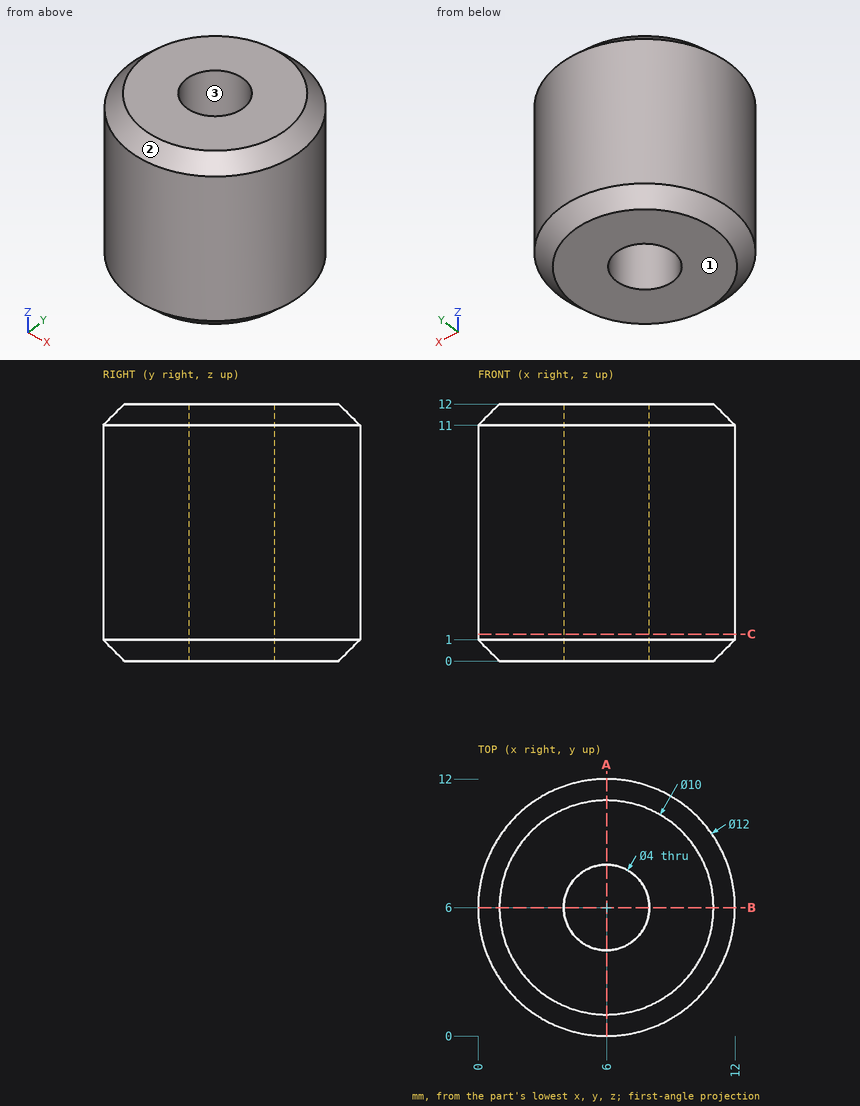
Study the drawing (mm; zero at the part's minimum x, y, z) and answer. Coordinates: 2 decimals unless noted, no trailing zeros. Loops run counter-clockwise (first coordinate to the right, second up) from the corner with the lowest first, then second, coordinate; pieces in that order, holes last. Notation, with made-up numbers: M 46,8 L 87,8 A16 ccw 87,17 Z; hole C -26.75,-38.75 d5. An arc over 180 degrees is marked long. Answer in a Markdown table with one row per item.
1) Determine the mould class of the marked faces 1, 2 and 3 for opening direction X: released by +X, released by -X, zero draft, split by the parting line, or undercut.
Answers below:
| item | result |
|---|---|
| face 1 | zero draft |
| face 2 | split by the parting line |
| face 3 | undercut |
2) Find section A-A (x = 6). Determine the outline of the cut face in (y, z), then the cut area to 3 significant figures.
Answers below:
| item | result |
|---|---|
| outline | M 0,1 L 1,0 L 4,0 L 4,12 L 1,12 L 0,11 Z; M 8,0 L 11,0 L 12,1 L 12,11 L 11,12 L 8,12 Z |
| area | 94.0 mm^2 |
3) Find section C-C (z = 1.25). Determine the outline of the cut face in (x, y), then the cut area to 3 significant figures.
Answers below:
| item | result |
|---|---|
| outline | C 6,6 d12; hole C 6,6 d4 |
| area | 101 mm^2 |
4) Find the intervals of material crossed by probe 1 along Y at (x, z) = (6, 7.75); probe 2 along X at (y, z) = (4.25, 9.25), in increasing order.
Answers below:
| item | result |
|---|---|
| probe 1 | 0 to 4, 8 to 12 |
| probe 2 | 0.26 to 5.03, 6.97 to 11.74 |
5) Given pin 1 (3 mm diameter, centred on y = 3.5, z = 1.5, fed in from -X); pin 2 (3.5 mm diameter, centred on x = 6, y = 6, fed in from -Z), each flat-ended and moving along its own axis, determine where each tip first touches the part or whether it passes through.
Answers below:
| item | result |
|---|---|
| pin 1 | x = 0.08 |
| pin 2 | through |
